The listing builds one solid part. Answer for the finished solid, in the listing's coordinates (mm). Face numbers are marked on the shaded views. A direction names the side the tool comes from. Round coordinates to 2 decimals unless told otherwise and drop trailing zeros. Write each loop counter-clockwise with the first axis right and the second up, starting at its lowest first coordinate (ties: lowest second). Pieces come first, ordered by that corner, then holes.
Item 1: Find the intervals of material crossed by probe 1 along Z at (x, y) = (-24, 10); probe 2 along X at (y, z) = (8.45, 5); probe 3 along Y at (x, z) = (18, 17), in increasing order.
Item 2: Find section B-B on x = 24. Give the vertices of the cut face in (y, z), then the cut area to 3 significant figures.
Item 3: Each of these flat-tipped pins is pushed along its axis until it touches: pin 1 (10 mm diameter, centred on y = -6.5, z = 13, fed in from -X); pin 2 (5.5 mm diameter, centred on y = 14, z = 7.5, fed in from +X); pin 3 (4 mm diameter, centred on x = 24, z = 15, fed in from +Y); pin 4 (6 mm diameter, centred on x = 10.5, z = 7.5, fed in from +Y). Where does it stop, or does it pass through?
Item 4: Find section D-D on x = -12. Give the vertices of the cut face in (y, z), then the cut area to 3 significant figures.
Item 5: A tool of negligible diameter and unlimited length cuts with its end or side. For the marked faces 1, 2, 3, 4 and 5, from which of +Z, -Z, +X, -X, +Y, -Y can it reach the whole face along a straight path? Write none if from no direction.
Item 6: Find section C-C on z = 2.5. Give the vertices of the cut face in (x, y), then the cut area to 3 significant figures.
Item 7: Find section A-A on z = 15. Give the vertices of the cut face in (x, y), then the cut area to 3 significant figures.
```python
from build123d import *

# Parameters (mm, degrees)
IZIM1_W                     = 40
IZIM1_H                     = 40
Y_KSEKLIK_EKSTR_ZYON1_DEPTH = 20
IZIM2_W                     = 20
IZIM2_H                     = 6
Y_KSEKLIK_EKSTR_ZYON2_DEPTH = 8
IZIM3_W                     = 20
IZIM3_H                     = 6
Y_KSEKLIK_EKSTR_ZYON3_DEPTH = 8
IZIM4_R                     = 2.5
Y_KSEKLIK_EKSTR_ZYON4_DEPTH = 5
IZIM5_R                     = 1.5
KES_EKSTR_ZYON1_DEPTH       = 15
RADYUS1_R                   = 1
RADYUS2_R                   = 1
RADYUS3_R                   = 1
RADYUS4_R                   = 1
RADYUS5_R                   = 1


with BuildPart() as part:
    # Çizim1 → Yükseklik-Ekstrüzyon1 (new body)
    with BuildSketch(Plane.XY):
        Rectangle(IZIM1_W, IZIM1_H)
    extrude(amount=Y_KSEKLIK_EKSTR_ZYON1_DEPTH)

    # Çizim2 → Yükseklik-Ekstrüzyon2 (add)
    with BuildSketch(Plane(origin=(20, 0, 0), x_dir=(0, 0, -1), z_dir=(1, 0, 0))):
        with Locations((-10, 9)):
            Rectangle(IZIM2_W, IZIM2_H)
    extrude(amount=Y_KSEKLIK_EKSTR_ZYON2_DEPTH)

    # Çizim3 → Yükseklik-Ekstrüzyon3 (add)
    with BuildSketch(Plane.ZY.offset(20)):
        with Locations((10, 9.60422947)):
            Rectangle(IZIM3_W, IZIM3_H)
    extrude(amount=Y_KSEKLIK_EKSTR_ZYON3_DEPTH)

    # Çizim4 → Yükseklik-Ekstrüzyon4 (add)
    with BuildSketch(Plane(origin=(0, 20, 0), x_dir=(1, 0, 0), z_dir=(0, 1, 0))):
        with Locations((-12, -10)):
            Circle(IZIM4_R)
    extrude(amount=Y_KSEKLIK_EKSTR_ZYON4_DEPTH)

    # Çizim5 → Kes-Ekstrüzyon1 (cut)
    with BuildSketch(Plane(origin=(0, 12.60422947, 0), x_dir=(1, 0, 0), z_dir=(0, 1, 0))):
        with Locations((-24, -5)):
            Circle(IZIM5_R)
        with Locations((-24, -15)):
            Circle(IZIM5_R)
        with Locations((24, -15)):
            Circle(IZIM5_R)
        with Locations((24, -5)):
            Circle(IZIM5_R)
    extrude(amount=-KES_EKSTR_ZYON1_DEPTH, mode=Mode.SUBTRACT)

    # Radyus1
    radyus1_edges = [part.edges().sort_by_distance(p)[0] for p in [
        (0, 20, 0),
        (-20, 20, 10),
        (20, 20, 10),
        (0, 20, 20),
    ]]
    fillet(radyus1_edges, radius=RADYUS1_R)

    # Radyus2
    radyus2_edges = [part.edges().sort_by_distance(p)[0] for p in [
        (0, -20, 20),
        (0, -20, 0),
        (20, -20, 10),
        (-20, -20, 10),
    ]]
    fillet(radyus2_edges, radius=RADYUS2_R)

    # Radyus3
    radyus3_edges = [part.edges().sort_by_distance(p)[0] for p in [
        (28, 9, 20),
    ]]
    fillet(radyus3_edges, radius=RADYUS3_R)

    # Radyus4
    radyus4_edges = [part.edges().sort_by_distance(p)[0] for p in [
        (-28, 9.60422947, 0),
    ]]
    fillet(radyus4_edges, radius=RADYUS4_R)

    # Radyus5
    radyus5_edges = [part.edges().sort_by_distance(p)[0] for p in [
        (28, 9, 0),
        (-28, 9.60422947, 20),
    ]]
    fillet(radyus5_edges, radius=RADYUS5_R)


solid = part.part
```
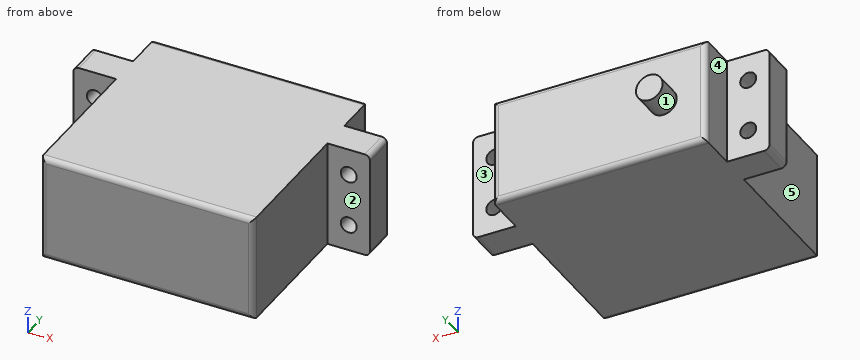
Check values:
1. probe 1: z = 0 to 3.5, 6.5 to 13.5, 16.5 to 20
1. probe 2: x = -28 to -25.5, -22.5 to 22.5, 25.5 to 28
1. probe 3: y = -20 to 20
2. outline: (6, 0) - (12, 0) - (12, 3.5) - (6, 3.5) - close; (6, 6.5) - (12, 6.5) - (12, 13.5) - (6, 13.5) - close; (6, 16.5) - (12, 16.5) - (12, 20) - (6, 20) - close
2. area: 84.0 mm2
3. pin 1: stops at x = -20
3. pin 2: stops at x = 28
3. pin 3: stops at y = 12
3. pin 4: stops at y = 20
4. outline: (-20, 1) arc R1 ccw to (-19, 0) - (19, 0) arc R1 ccw to (20, 1) - (20, 7.5) - (25, 7.5) - (25, 12.5) - (20, 12.5) - (20, 19) arc R1 ccw to (19, 20) - (-19, 20) arc R1 ccw to (-20, 19) - close
4. area: 824 mm2
5. face 1: +Y
5. face 2: +Z, -Z, +X, -Y
5. face 3: +Z, -Z, +X, +Y
5. face 4: +Z, -Z, -X, +Y
5. face 5: +Z, -Z, -X, -Y
6. outline: (-28, 6.6) - (-20, 6.6) - (-20, -19) arc R1 ccw to (-19, -20) - (19, -20) arc R1 ccw to (20, -19) - (20, 6) - (28, 6) - (28, 12) - (20, 12) - (20, 19) arc R1 ccw to (19, 20) - (-19, 20) arc R1 ccw to (-20, 19) - (-20, 12.6) - (-28, 12.6) - close
6. area: 1,700 mm2
7. outline: (-28, 6.6) - (-25.5, 6.6) - (-25.5, 12.6) - (-28, 12.6) - close; (-22.5, 6.6) - (-20, 6.6) - (-20, -19) arc R1 ccw to (-19, -20) - (19, -20) arc R1 ccw to (20, -19) - (20, 6) - (22.5, 6) - (22.5, 12) - (20, 12) - (20, 19) arc R1 ccw to (19, 20) - (-19, 20) arc R1 ccw to (-20, 19) - (-20, 12.6) - (-22.5, 12.6) - close; (25.5, 6) - (28, 6) - (28, 12) - (25.5, 12) - close
7. area: 1,660 mm2
